Verification items for the finished model (mm, model axes). A direction names the side the tool comes from. Coordinates: 2 decimals unless noted, no trailing zeros. Order: outer loops, then holes, each group sorted by start corner. A loop starts at its lowest first (then second) coordinate and runs counter-clockwise, first axis right, second up. Notation, with made-up numbers: (48, 54) -> (104, 54) arc R21 cw to (104, 89) -> close; hole circle Ø1 at (-36, 66). An arc over 180 degrees is marked (long way). Write item = value, one per line. Start each with the question number.
from build123d import *

# Parameters (mm, degrees)
BOSS_EXTRUDE1_DEPTH = 5
CUT_EXTRUDE1_DEPTH  = 3
SKETCH3_W           = 9
SKETCH3_H           = 10
SKETCH3_R           = 1.5
BOSS_EXTRUDE2_DEPTH = 2


with BuildPart() as part:
    # Sketch1 → Boss-Extrude1 (new body, symmetric)
    with BuildSketch(Plane(origin=(0, 0, 0), x_dir=(1, 0, 0), z_dir=(0, 1, 0))):
        with BuildLine():
            Line((5.715, 0), (12.7, 0))
            ThreePointArc((12.7, 0), (0, 12.7), (-12.7, 0))
            Line((-12.7, 0), (-5.715, 0))
            ThreePointArc((-5.715, 0), (0, 5.715), (5.715, 0))
        make_face()
    extrude(amount=BOSS_EXTRUDE1_DEPTH, both=True)

    # Sketch2 → Cut-Extrude1 (cut, symmetric)
    with BuildSketch(Plane(origin=(0, 0, 0), x_dir=(1, 0, 0), z_dir=(0, 1, 0))):
        with BuildLine():
            ThreePointArc((6.985, 0), (0, 6.985), (-6.985, 0))
            Line((-6.985, 0), (6.985, 0))
        make_face()
        with BuildLine():
            Line((6.985, 0), (-6.985, 0))
            ThreePointArc((-6.985, 0), (0, -6.985), (6.985, 0))
        make_face()
    extrude(amount=CUT_EXTRUDE1_DEPTH, both=True, mode=Mode.SUBTRACT)

    # Sketch3 → Boss-Extrude2 (add)
    with BuildSketch(Plane.XY):
        with Locations((15.5, 0)):
            Rectangle(SKETCH3_W, SKETCH3_H)
        with Locations((15, 0)):
            Circle(SKETCH3_R, mode=Mode.SUBTRACT)
        with Locations((-15.5, 0)):
            Rectangle(SKETCH3_W, SKETCH3_H)
        with Locations((-15, 0)):
            Circle(SKETCH3_R, mode=Mode.SUBTRACT)
    extrude(amount=-BOSS_EXTRUDE2_DEPTH)


solid = part.part
Item 1: Thickness scan on line 1 (Y direction, x = 15, z = -1.15); line 2 (Z direction, x = 14, y = -2.75); line 3 (X direction, y = -1.5, z = -4.75). Record the ranges inside material, lowest first.
Item 2: Section check A-A (z = -0.75). Record the boundary of the cut face in (x, y), then the cut area to 3 significant figures.
Item 3: Mould release check, pull along X, two halves, no side actions. Record for faces 1 (the flat face through (13, 0, 0)), 2 (the cylindrical face through (-0.126, 4.014, -5.714)), 3 (the flat face through (-20, 0, -1)), 4 (the flat face through (-1, -3, -6)): pulls with the +X half, pulls with the -X half, needs draft (parallel to the pull), parting line crosses it, or undercut.
Item 4: Gauge pin test, flat ends, axial feed: P1, Ø5, axis at y = 3, z = -10.5, coming from the -X side; P2, Ø1, axis at x = -2.5, z = -3.5, coming from the -Y side; P3, Ø3.5, axis at x = 15, y = 0, coming from the -Z side; P4, Ø6, axis at y = 4, z = -10, coming from the -X side. Record the tip position at first contact, or that the pin passes through.
Item 5: Tool access check on faces 5 (the flat face through (-17, 0, -2)), 6 (the cylindrical face through (0.154, 0.042, -6.983)), 7 (the flat face through (17, 0, -2)). Record the directions out of +Z, -Z, +X, -X, +Y, -Y that give a thin tool (end or side, any length) a straight path to the whole face; none if there is none.
Item 6: Section check D-D (y = 4). Record the boundary of the cut face in (x, z) (3 decimals), then the cut area to 3 significant figures.
Item 7: Section check B-B (y = 0). Record the boundary of the cut face in (x, z) (3 decimals).
Item 8: Section check C-C (x = -15). Record the boundary of the cut face in (y, z).
Filled sheet:
q1.line_1 = -5 to -1.5, 1.5 to 5
q1.line_2 = -2 to 0
q1.line_3 = -11.78 to -5.12, 5.12 to 11.78
q2.outline = (-20, -5) -> (-5.67, -5) -> (-5.67, -3) -> (-6.94, -3) -> (-6.94, 3) -> (-5.67, 3) -> (-5.67, 5) -> (-20, 5) -> close; (5.67, -5) -> (20, -5) -> (20, 5) -> (5.67, 5) -> (5.67, 3) -> (6.94, 3) -> (6.94, -3) -> (5.67, -3) -> close; hole circle Ø3 at (-15, 0); hole circle Ø3 at (15, 0)
q2.area = 257 mm^2
q3.face_1 = needs draft
q3.face_2 = undercut
q3.face_3 = pulls with the -X half
q3.face_4 = undercut
q4.P1 = -9.86
q4.P2 = through
q4.P3 = -2
q4.P4 = -10.6
q5.face_5 = -Z, -X, +Y, -Y
q5.face_6 = +Z
q5.face_7 = -Z, +X, +Y, -Y
q6.outline = (-20, -2) -> (-12.542, -2) arc R12.7 ccw to (12.542, -2) -> (20, -2) -> (20, 0) -> (5.715, 0) arc R5.715 cw to (-5.715, 0) -> (-20, 0) -> close
q6.area = 231 mm^2
q7.outline = (-20, -2) -> (-16.5, -2) -> (-16.5, 0) -> (-20, 0) -> close; (-13.5, -2) -> (-12.542, -2) arc R12.7 ccw to (12.542, -2) -> (13.5, -2) -> (13.5, 0) -> (6.985, 0) arc R6.985 cw to (-6.985, 0) -> (-13.5, 0) -> close; (16.5, -2) -> (20, -2) -> (20, 0) -> (16.5, 0) -> close
q8.outline = (-5, -2) -> (-1.5, -2) -> (-1.5, 0) -> (-5, 0) -> close; (1.5, -2) -> (5, -2) -> (5, 0) -> (1.5, 0) -> close
